Autodesk Inventor part; units mm, degrees
ref_plane "YZ Plane" through (0, 0, 0) normal (1, 0, 0) x (0, 1, 0)
ref_plane "XZ Plane" through (0, 0, 0) normal (0, 1, 0) x (-1, 0, 0)
ref_plane "XY Plane" through (0, 0, 0) normal (0, 0, 1) x (1, 0, 0)
sketch "Sketch1" plane through (0, 0, 0) normal (0, 0, 1) x (1, 0, 0)
  circle A0 centre (47, 53.101) radius 5.025
  line L0 (47, 53.101) -> (61.1421, 67.2432) construction
  circle A1 centre (61.1421, 67.2432) radius 5.025
  circle A2 centre (61.1421, 67.2432) radius 9.5
  circle A3 centre (47, 53.101) radius 8.5
  line L1 (68.5668, 88.1028) -> (54.4246, 73.9607)
  arc A4 (74.5933, 82.8719) -> (68.5668, 88.1028) centre (71.3952, 85.2744) ccw
  arc A5 (74.5933, 82.8719) -> (75.0285, 70.3201) centre (82.5886, 76.8657) ccw
  arc A6 (74.9307, 67.5967) -> (75.0285, 70.3201) centre (73.5165, 69.0109) ccw
  line L2 (74.9307, 67.5967) -> (67.8597, 60.5257)
  circle A7 centre (47, 53.101) radius 7.5
  circle A8 centre (61.1421, 67.2432) radius 7.5
  arc A9 (42.6661, 60.4132) -> (52.5446, 71.2845) centre (29.9195, 81.9195) ccw
  arc A10 (64.4883, 58.352) -> (54.6431, 49.3817) centre (70.8284, 41.5055) ccw
  line L3 (124.9643, 38.1784) -> (101.7414, 38.1784) construction
  point P0 (0, 0)
  dimension "d33" = 10.05
  dimension "d34" = 20
  dimension "d35" = 10.05
  dimension "d36" = 19
  dimension "d37" = 17
  dimension "d38" = 4
  dimension "d39" = 2
  dimension "d40" = 10
  dimension "d41" = 20
  dimension "d42" = 10
  dimension "d43" = 15
  dimension "d44" = 15
  dimension "d45" = 25
  dimension "d46" = 18
  dimension "d47" = 45
extrude "Extrusion1" add sketch "Sketch1" against normal blind 3 contours A2 | A2 L1 A4 A5 A6 L2 | A2 A10 A3 A9 | A3 | A7
extrude "Extrusion2" add sketch "Sketch1" against normal blind 2 contours A8
properties part number "dsa" material "Aluminum 7075"
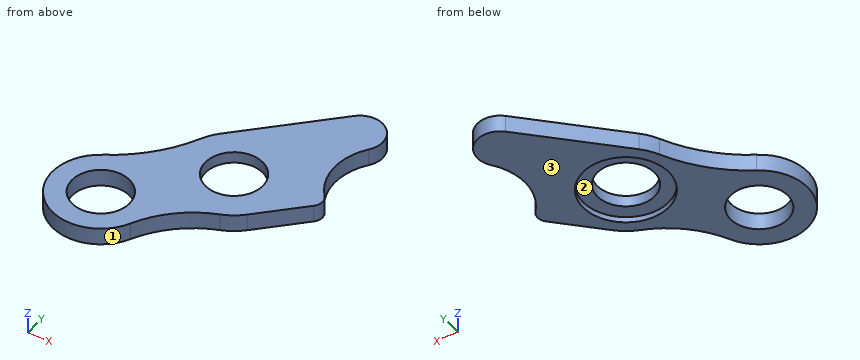
Check sheet for the modelled part. Datum: model origin and axes. Units: mm. Face numbers are marked on the shaded views. Round coordinates to 2 decimals unless told otherwise and drop trailing zeros. Loops run counter-clockwise (first coordinate to the right, second up) from the corner with the lowest first, then second, coordinate; pieces in that order, holes last. Notation, with made-up numbers: M -13.5,57 L 18.5,57 A22 cw 18.5,94 Z; hole C 73.25,-37.5 d4. An arc over 180 degrees is marked long. One line per item, written item: value.
(1) Sectioned sample at D-D, the plane x = 59. Record the cut outline in (y, z).
Computed values:
outline: M 55.07,-3 L 60.06,-3 L 60.06,-2 L 62.7,-2 L 62.7,0 L 55.07,0 Z; M 71.79,-2 L 74.43,-2 L 74.43,-3 L 78.54,-3 L 78.54,0 L 71.79,0 Z
(2) Sectioned sample at A-A, the plane x = 47. Record the cut outline in (y, z).
Computed values:
outline: M 44.6,-3 L 48.08,-3 L 48.08,0 L 44.6,0 Z; M 58.13,-3 L 63.66,-3 L 63.66,0 L 58.13,0 Z
(3) Sectioned sample at B-B, the plane y = 56.5. Record the cut outline in (x, z).
Computed values:
outline: M 39.21,-3 L 43.3,-3 L 43.3,0 L 39.21,0 Z; M 50.7,-3 L 60.87,-3 L 60.87,0 L 50.7,0 Z
(4) Depth check by flat-ended pin: pin 1 Ø1.5 at (y, z) = (55.5, -1.5) entering from -X; pin 2 Ø7.5 at (x, y) = (60.5, 65) entering from -Z; pin 3 Ø1.5 at (y, z) = (77.5, -2) entering from +X; pin 4 Ø10 at (x, y) = (43, 52.5) entering from +Z. Enter the tip coordinate at first touch or a pass-through.
Computed values:
pin 1: stops at x = 38.66
pin 2: stops at z = -2
pin 3: stops at x = 72.68
pin 4: stops at z = 0
(5) Sectioned sample at C-C, the plane z = -1.05. Count the separate pieces of the cut face and the enclosed holes in it, then the cut area to 3 significant figures.
Computed values:
separate pieces: 1
enclosed holes: 2
area: 613 mm^2
(6) Release check for a two-part mould opening along X. For the marked faces 1, 2 and 3 record: +X half, -X half, draft (parallel to the pull), parting line (faces both ways), or undercut.
Computed values:
face 1: parting line
face 2: undercut
face 3: draft
(7) Thickness scan on line 1 (Y direction, x = 47.5, z = -0.4); line 2 (Y direction, x = 44, z = -1.1); line 3 (X direction, y = 49, z = -0.25). Record the ranges inside material, lowest first.
Computed values:
line 1: y = 44.62 to 48.1, 58.1 to 64.15
line 2: y = 45.15 to 49.07, 57.13 to 61.26
line 3: x = 39.55 to 44.1, 49.9 to 54.45
